from build123d import *

# Parameters (mm, degrees)
BOSS_EXTRUDE1_DEPTH  = 4.7625
M4_CLEARANCE_HOLE1_D = 4.5
SKETCH4_R            = 3.3
SKETCH4_R_2          = 2.9765625
SKETCH4_R_3          = 6.445
SKETCH4_R_4          = 11.9
CUT_EXTRUDE1_DEPTH   = 4.7625
BOSS_EXTRUDE3_DEPTH  = 4.7625
M4_CLEARANCE_HOLE2_D = 4.5


with BuildPart() as part:
    # Sketch1 → Boss-Extrude1 (new body)
    with BuildSketch(Plane.XY):
        with BuildLine():
            Line((50.349976536, 7.779015878), (19.528151129, 7.779015878))
            Line((19.528151129, 7.779015878), (16.547693582, 10.759473425))
            ThreePointArc((16.547693582, 10.759473425), (8.769518989, 10.759473425), (8.769518989, 2.981298831))
            Line((8.769518989, 2.981298831), (11.749976536, 0.000841285))
            Line((11.749976536, 0.000841285), (11.749976536, -43.901984122))
            Line((11.749976536, -43.901984122), (8.340276536, -43.901984122))
            ThreePointArc((8.340276536, -43.901984122), (2.840276536, -49.401984122), (8.340276536, -54.901984122))
            Line((8.340276536, -54.901984122), (11.749976536, -54.901984122))
            Line((11.749976536, -54.901984122), (11.749976536, -100.289984122))
            Line((11.749976536, -100.289984122), (8.340276536, -100.289984122))
            ThreePointArc((8.340276536, -100.289984122), (2.840276536, -105.789984122), (8.340276536, -111.289984122))
            Line((8.340276536, -111.289984122), (11.749976536, -111.289984122))
            Line((11.749976536, -111.289984122), (11.749976536, -155.192809529))
            Line((11.749976536, -155.192809529), (8.769518989, -158.173267075))
            ThreePointArc((8.769518989, -158.173267075), (8.769518989, -165.951441668), (16.547693582, -165.951441668))
            Line((16.547693582, -165.951441668), (19.528151129, -162.970984122))
            Line((19.528151129, -162.970984122), (50.349976536, -162.970984122))
            Line((50.349976536, -162.970984122), (50.349976536, -166.380684122))
            ThreePointArc((50.349976536, -166.380684122), (55.849976536, -171.880684122), (61.349976536, -166.380684122))
            Line((61.349976536, -166.380684122), (61.349976536, -162.970984122))
            Line((61.349976536, -162.970984122), (92.171801943, -162.970984122))
            Line((92.171801943, -162.970984122), (95.152259489, -165.951441668))
            ThreePointArc((95.152259489, -165.951441668), (102.930434082, -165.951441668), (102.930434082, -158.173267075))
            Line((102.930434082, -158.173267075), (99.949976536, -155.192809529))
            Line((99.949976536, -155.192809529), (99.949976536, -111.289984122))
            Line((99.949976536, -111.289984122), (103.359676536, -111.289984122))
            ThreePointArc((103.359676536, -111.289984122), (108.859676536, -105.789984122), (103.359676536, -100.289984122))
            Line((103.359676536, -100.289984122), (99.949976536, -100.289984122))
            Line((99.949976536, -100.289984122), (99.949976536, -54.901984122))
            Line((99.949976536, -54.901984122), (103.359676536, -54.901984122))
            ThreePointArc((103.359676536, -54.901984122), (108.859676536, -49.401984122), (103.359676536, -43.901984122))
            Line((103.359676536, -43.901984122), (99.949976536, -43.901984122))
            Line((99.949976536, -43.901984122), (99.949976536, 0.000841285))
            Line((99.949976536, 0.000841285), (102.930434082, 2.981298831))
            ThreePointArc((102.930434082, 2.981298831), (102.930434082, 10.759473425), (95.152259489, 10.759473425))
            Line((95.152259489, 10.759473425), (92.171801943, 7.779015878))
            Line((92.171801943, 7.779015878), (61.349976536, 7.779015878))
            Line((61.349976536, 7.779015878), (61.349976536, 11.188715878))
            ThreePointArc((61.349976536, 11.188715878), (55.849976536, 16.688715878), (50.349976536, 11.188715878))
            Line((50.349976536, 11.188715878), (50.349976536, 7.779015878))
        make_face()
    extrude(amount=-BOSS_EXTRUDE1_DEPTH)

    # M4 Clearance Hole1 (through all)
    with Locations(Plane(origin=(0, 0, -4.7625), x_dir=(-1, 0, 0), z_dir=(0, 0, -1))):
        with Locations((-12.658606286, -162.062354372), (-55.849976536, -166.380684122), (-99.041346785, -162.062354372), (-103.359676536, -105.789984122), (-103.359676536, -49.401984122), (-99.041346785, 6.870386128), (-12.658606286, 6.870386128), (-8.340276536, -49.401984122), (-8.340276536, -105.789984122), (-55.849976536, 11.188715878)):
            Hole(M4_CLEARANCE_HOLE1_D / 2)

    # Sketch4 → Cut-Extrude1 (cut)
    with BuildSketch(Plane(origin=(0, 0, -4.7625), x_dir=(-1, 0, 0), z_dir=(0, 0, -1))):
        with Locations((-41.616084767, -16.665859852)):
            Circle(SKETCH4_R)
        with Locations((-70.083868304, -40.3002691)):
            Circle(SKETCH4_R)
        with Locations((-27.909976536, -139.508484122)):
            Circle(SKETCH4_R_2)
        with Locations((-41.616084767, -76.466699143)):
            Circle(SKETCH4_R)
        with Locations((-83.789976536, -139.508484122)):
            Circle(SKETCH4_R_2)
        with Locations((-70.083868304, -100.101108391)):
            Circle(SKETCH4_R)
        with Locations((-66.009976536, -139.508484122)):
            Circle(SKETCH4_R_3)
        with Locations((-82.519976536, -59.220984122)):
            Circle(SKETCH4_R_3)
        with Locations((-45.689976536, -139.508484122)):
            Circle(SKETCH4_R_3)
        with Locations((-55.849976536, -88.283903767)):
            Circle(SKETCH4_R_4)
        with Locations((-55.849976536, -28.483064476)):
            Circle(SKETCH4_R_4)
    extrude(amount=-CUT_EXTRUDE1_DEPTH, mode=Mode.SUBTRACT)

    # Sketch6 → Boss-Extrude3 (add)
    with BuildSketch(Plane.XY):
        with BuildLine():
            Line((39.939063832, 7.779015878), (39.939063832, 12.779015878))
            ThreePointArc((39.939063832, 12.779015878), (34.939063832, 17.779015878), (29.939063832, 12.779015878))
            Line((29.939063832, 12.779015878), (29.939063832, 7.779015878))
            Line((29.939063832, 7.779015878), (39.939063832, 7.779015878))
        make_face()
        with BuildLine():
            Line((81.760889239, -162.970984122), (71.760889239, -162.970984122))
            Line((71.760889239, -162.970984122), (71.760889239, -167.970984122))
            ThreePointArc((71.760889239, -167.970984122), (76.760889239, -172.970984122), (81.760889239, -167.970984122))
            Line((81.760889239, -167.970984122), (81.760889239, -162.970984122))
        make_face()
    boss_extrude3 = extrude(amount=-BOSS_EXTRUDE3_DEPTH)

    # M4 Clearance Hole2 (through all)
    with Locations(Plane.XY):
        with Locations((34.939063832, 12.779015878), (76.760889239, -167.970984122)):
            m4_clearance_hole2 = Hole(M4_CLEARANCE_HOLE2_D / 2)

    # Mirror1: Boss-Extrude3, M4 Clearance Hole2 across plane
    add(boss_extrude3.mirror(Plane.ZY.offset(-55.849976536)))
    add(m4_clearance_hole2.mirror(Plane.ZY.offset(-55.849976536)), mode=Mode.SUBTRACT)


solid = part.part
Could you check a few things on this model? Use its own coordinates, in mm. A direction names the side the tool comes from. Round coordinates to 2 decimals unless told otherwise and drop trailing zeros. Order: outer loops, then holes, each group sorted by start corner. A loop starts at its lowest first (then second) coordinate and runs counter-clockwise, first axis right, second up.
(1) Imagine slicing it at B-B (x = 84.5). Write out the boundary of the cut face in (y, z), plus the area to 3 significant figures.
Response values:
outline: (-162.97, -4.76) - (-142.4, -4.76) - (-142.4, 0) - (-162.97, 0) - close; (-136.62, -4.76) - (-65.35, -4.76) - (-65.35, 0) - (-136.62, 0) - close; (-53.09, -4.76) - (7.78, -4.76) - (7.78, 0) - (-53.09, 0) - close
area: 727 mm2
(2) Please list where these lines run through material, in increasing order: line 1 along X through (y, z) = (7, -0.2); line 2 along Y through (x, z) = (102.5, -0.35); line 3 along Y through (x, z) = (51, -1).
Response values:
line 1: x = 7.16 to 10.41, 14.9 to 96.8, 101.29 to 104.54
line 2: y = -166.34 to -157.74, -111.29 to -107.87, -103.71 to -100.29, -54.9 to -51.48, -47.32 to -43.9, 2.55 to 11.15
line 3: y = -168.97 to -143.16, -135.86 to -99.15, -77.42 to -39.35, -17.62 to 13.78
(3) Which directions (+Z, -Z, +X, -X, +Y, -Y) give clear straight access to the entire face, cutting with the end or side of a thin tool? Please do faces 1 (the flat face through (45, -162.971, -2)), 2 (the flat face through (67, 7.779, -2)), 3 (the cylindrical face through (108.86, -49.52, -2.35)), 4 (the flat face through (10, -43.902, -2)), 5 (the cylindrical face through (50.36, -98.84, -2.41)).
Response values:
face 1: +Z, -Z, -Y
face 2: +Z, -Z, +Y
face 3: +Z, -Z, +X
face 4: +Z, -Z, -X
face 5: +Z, -Z
(4) I'm going to push flat-ended pins straight in: pin 1 (2.5 mm diameter, centred on x = 11, z = -3, fed in from +Y); pin 2 (7.5 mm diameter, centred on x = 66.01, y = -139.51, fed in from +Z); pin 3 (1 mm diameter, centred on x = 39, z = -3.5, fed in from +Y); pin 4 (8.5 mm diameter, centred on x = 41.62, y = -76.47, fed in from +Z). Where does each tip first touch, or does it pass through?
Response values:
pin 1: stops at y = 12.36
pin 2: passes through
pin 3: stops at y = 16.29
pin 4: stops at z = 0
(5) If we mould it in two halves opening along X, with no side actions, what happens to faces 6 (the flat face through (10, -111.29, -2)), 7 (the flat face through (87, 7.779, -2)), 8 (the cylindrical face through (2.84, -105.67, -2.35))? For each: released by +X, released by -X, zero draft, split by the parting line, or undercut.
Response values:
face 6: zero draft
face 7: undercut
face 8: released by -X
(6) Imagine slicing it at A-A (x = 64.5). Write out the boundary of the cut face in (y, z).
Response values:
outline: (-162.97, -4.76) - (-145.77, -4.76) - (-145.77, 0) - (-162.97, 0) - close; (-133.24, -4.76) - (-96.46, -4.76) - (-96.46, 0) - (-133.24, 0) - close; (-80.11, -4.76) - (-36.66, -4.76) - (-36.66, 0) - (-80.11, 0) - close; (-20.31, -4.76) - (7.78, -4.76) - (7.78, 0) - (-20.31, 0) - close
(7) Imagine slicing it at C-C (y = -129.5). Write out the boundary of the cut face in (x, z), plus the area to 3 significant figures.
Response values:
outline: (11.75, -4.76) - (99.95, -4.76) - (99.95, 0) - (11.75, 0) - close
area: 420 mm2
(8) Imagine slicing it at D-D (z = -3.25). Count the separate pieces of the cut face and the enclosed holes in it, plus the area to 3 significant figures.
Response values:
separate pieces: 1
enclosed holes: 25
area: 14,500 mm2
